Could you check a few things on this model? Use its own coordinates, in mm. Coordinates: 2 decimals unless noted, no trailing zeros. Write each loop counter-clockwise with the first axis right and the second up, starting at its lowest first coordinate (ties: lowest second). Pieces come first, ordered by that corner, then holes. Notation, with made-up numbers: M 22,-33 L 41,-33 A25 ccw 41,5 Z; hole C -22,15.25 d10. An arc over 180 degrees is marked long. Answer as CSV lines item,"result". Start each with the question number.
Item 1: I'm going to push flat-ended pins straight in: P1, Ø4, axis at x = -29.5, z = 70, coming from the -Y side; P2, Ø7.5, axis at x = -69, y = 13, coming from the -Z side; P3, Ø7.5, axis at x = 14, y = 79.5, coming from the +Z side. Where does each tip first touch, or does it pass through?
Item 2: Suppose I cut it at A-A, the plane x = -63. Write out the boundary of the cut face in (y, z).
Item 3: Suppose I cut it at C-C, the plane y = 90. Write out the boundary of the cut face in (x, z).
Item 4: If I drill on line 1 along Y through (x, z) = (-88, 689.5); line 2 along X through (y, z) = (25, 433); line 3 along X through (y, z) = (32.5, 429.5), over which ranges is the centre line in solid material (lowest first)? Write a range as [from, to].
Item 5: Suppose I cut it at B-B, the plane y = -90. Write out the boundary of the cut face in (x, z).
Item 6: Suppose I cut it at D-D, the plane z = 653. Write out the boundary of the cut face in (x, y).
```python
from build123d import *

# Parameters (mm, degrees)
SKETCH_1_R           = 49
EXTRUDE_1_DEPTH      = 800
SKETCH_6_W           = 80
SKETCH_6_H           = 50
EXTRUDE_4_DEPTH      = 120
SKETCH_7_W           = 79.068992587
SKETCH_7_H           = 50.572115984
EXTRUDE_5_DEPTH      = 120
SKETCH_8_W           = 50
SKETCH_8_H           = 80
EXTRUDE_6_DEPTH      = 120
SKETCH_11_W          = 50
SKETCH_11_H          = 80
EXTRUDE_7_DEPTH      = 240
SKETCH_12_W          = 81
SKETCH_12_H          = 20
CUT_EXTRUDE_2_DEPTH  = 240
SKETCH_13_W          = 0.776791224
SKETCH_13_H          = 19.974152477
CUT_EXTRUDE_3_DEPTH  = 240
SKETCH_14_W          = 20
SKETCH_14_H          = 80
CUT_EXTRUDE_4_DEPTH  = 240
SKETCH_15_R          = 10
CUT_EXTRUDE_5_DEPTH  = 240
SKETCH_16_R          = 10
CUT_EXTRUDE_7_DEPTH  = 240
SKETCH_17_R          = 10
CUT_EXTRUDE_8_DEPTH  = 240
SKETCH_18_R          = 10
CUT_EXTRUDE_9_DEPTH  = 240
SKETCH_20_R          = 49
EXTRUDE_11_DEPTH     = 600
SKETCH_19_R          = 37.31025629
CUT_EXTRUDE_10_DEPTH = 818.80193201
CUT_EXTRUDE_START    = -600
SKETCH_21_R          = 49
CUT_EXTRUDE_11_DEPTH = 600
EXTRUDE_START        = 600
SKETCH_22_R          = 49
EXTRUDE_12_DEPTH     = 600
SKETCH_23_R          = 49
CUT_EXTRUDE_13_DEPTH = 500


with BuildPart() as part:
    # 草图1 → 凸台-拉伸1 (new body)
    with BuildSketch(Plane.XY):
        Circle(SKETCH_1_R)
    extrude(amount=EXTRUDE_1_DEPTH)

    # 草图6 → 凸台-拉伸4 (add)
    with BuildSketch(Plane(origin=(0, 0, 0), x_dir=(0, 0, -1), z_dir=(1, 0, 0))):
        with Locations((-729.062639013, -6.734256512)):
            Rectangle(SKETCH_6_W, SKETCH_6_H)
    extrude(amount=EXTRUDE_4_DEPTH)

    # 草图7 → 凸台-拉伸5 (add)
    with BuildSketch(Plane(origin=(0, 0, 0), x_dir=(0, 0, -1), z_dir=(1, 0, 0))):
        with Locations((-728.814319263, -6.902168752)):
            Rectangle(SKETCH_7_W, SKETCH_7_H)
    extrude(amount=-EXTRUDE_5_DEPTH)

    # 草图8 → 凸台-拉伸6 (add)
    with BuildSketch(Plane(origin=(0, 0, 0), x_dir=(1, 0, 0), z_dir=(0, 1, 0))):
        with Locations((0, -728.037522505)):
            Rectangle(SKETCH_8_W, SKETCH_8_H)
    extrude(amount=EXTRUDE_6_DEPTH)

    # 草图11 → 凸台-拉伸7 (add)
    with BuildSketch(Plane(origin=(0, 120, 0), x_dir=(1, 0, 0), z_dir=(0, 1, 0))):
        with Locations((0, -728.408363968)):
            Rectangle(SKETCH_11_W, SKETCH_11_H)
    extrude(amount=-EXTRUDE_7_DEPTH)

    # 草图12 → 切除-拉伸2 (cut)
    with BuildSketch(Plane.ZY.offset(120)):
        with Locations((727.848815556, -6.61611076)):
            Rectangle(SKETCH_12_W, SKETCH_12_H)
    extrude(amount=-CUT_EXTRUDE_2_DEPTH, mode=Mode.SUBTRACT)

    # 草图13 → 切除-拉伸3 (cut)
    with BuildSketch(Plane(origin=(120, 0, 0), x_dir=(0, 0, -1), z_dir=(1, 0, 0))):
        with Locations((-768.737211168, -6.577297247)):
            Rectangle(SKETCH_13_W, SKETCH_13_H)
    extrude(amount=-CUT_EXTRUDE_3_DEPTH, mode=Mode.SUBTRACT)

    # 草图14 → 切除-拉伸4 (cut)
    with BuildSketch(Plane(origin=(0, -120, 0), x_dir=(-1, 0, 0), z_dir=(0, -1, 0))):
        with Locations((0, -728.408363968)):
            Rectangle(SKETCH_14_W, SKETCH_14_H)
    extrude(amount=-CUT_EXTRUDE_4_DEPTH, mode=Mode.SUBTRACT)

    # 草图15 → 切除-拉伸5 (cut)
    with BuildSketch(Plane(origin=(0, 18.38388924, 0), x_dir=(1, 0, 0), z_dir=(0, 1, 0))):
        with Locations(Location((-90, -729.279822969, 0), (0, 0, 270))):
            Circle(SKETCH_15_R)
    extrude(amount=-CUT_EXTRUDE_5_DEPTH, mode=Mode.SUBTRACT)

    # 草图16 → 切除-拉伸7 (cut)
    with BuildSketch(Plane.ZY.offset(25)):
        with Locations((728.037522505, 90)):
            Circle(SKETCH_16_R)
    extrude(amount=-CUT_EXTRUDE_7_DEPTH, mode=Mode.SUBTRACT)

    # 草图17 → 切除-拉伸8 (cut)
    with BuildSketch(Plane(origin=(0, 18.265743488, 0), x_dir=(1, 0, 0), z_dir=(0, 1, 0))):
        with Locations(Location((90, -729.062639013, 0), (0, 0, 270))):
            Circle(SKETCH_17_R)
    extrude(amount=-CUT_EXTRUDE_8_DEPTH, mode=Mode.SUBTRACT)

    # 草图18 → 切除-拉伸9 (cut)
    with BuildSketch(Plane(origin=(25, 0, 0), x_dir=(0, 0, -1), z_dir=(1, 0, 0))):
        with Locations((-728.408363968, -90)):
            Circle(SKETCH_18_R)
    extrude(amount=-CUT_EXTRUDE_9_DEPTH, mode=Mode.SUBTRACT)

    # 草图20 → 凸台-拉伸11 (add)
    with BuildSketch(Plane.XY.offset(800)):
        Circle(SKETCH_20_R)
    extrude(amount=EXTRUDE_11_DEPTH)

    # 草图19 → 切除-拉伸10 (cut, through all)
    with BuildSketch(Plane.XY.offset(800)):
        Circle(SKETCH_19_R)
    extrude(amount=CUT_EXTRUDE_10_DEPTH, mode=Mode.SUBTRACT)

    # 草图21 → 切除-拉伸11 (cut)
    with BuildSketch(Plane.XY.offset(1400).offset(CUT_EXTRUDE_START)):
        Circle(SKETCH_21_R)
    extrude(amount=CUT_EXTRUDE_11_DEPTH, mode=Mode.SUBTRACT)

    # 草图22 → 凸台-拉伸12 (add)
    with BuildSketch(Plane(origin=(0, 0, 0), x_dir=(-1, 0, 0), z_dir=(0, 0, -1)).offset(EXTRUDE_START)):
        Circle(SKETCH_22_R)
    extrude(amount=-EXTRUDE_12_DEPTH)

    # 草图23 → 切除-拉伸13 (cut)
    with BuildSketch(Plane(origin=(0, 0, -600), x_dir=(-1, 0, 0), z_dir=(0, 0, -1))):
        Circle(SKETCH_23_R)
    extrude(amount=-CUT_EXTRUDE_13_DEPTH, mode=Mode.SUBTRACT)


solid = part.part
```
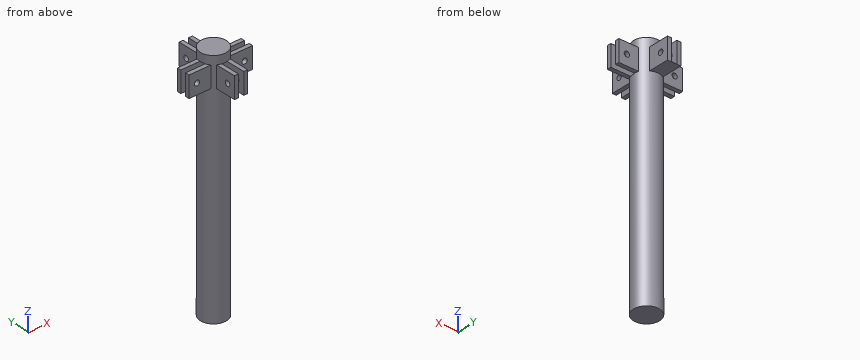
Ans:
1,P1,"stops at y = -40.56"
1,P2,"stops at z = 689.28"
1,P3,"stops at z = 768.41"
2,outline,"M -32.19,689.28 L -16.62,689.28 L -16.62,768.35 L -32.19,768.35 Z; M 3.38,689.28 L 18.38,689.28 L 18.38,768.35 L 3.38,768.35 Z"
3,outline,"M -25,688.04 L 25,688.04 L 25,718.04 L 10,718.04 L 10,688.41 L -10,688.41 L -10,718.04 L -25,718.04 Z; M -25,738.04 L -10,738.04 L -10,768.41 L -25,768.41 Z; M 10,738.04 L 25,738.04 L 25,768.41 L 10,768.41 Z"
4,line 1,"y = [-32.19, -16.62], [3.38, 18.38]"
4,line 2,"x = [-42.14, 42.14]"
4,line 3,"x = [-36.67, 36.67]"
5,outline,"M -25,688.41 L -10,688.41 L -10,718.41 L -25,718.41 Z; M -25,738.41 L -10,738.41 L -10,768.41 L -25,768.41 Z; M 10,688.41 L 25,688.41 L 25,718.41 L 10,718.41 Z; M 10,738.41 L 25,738.41 L 25,768.41 L 10,768.41 Z"
6,outline,"C 0,0 d98"
